Source: CAD feature listing. Evaluate the final solid. Frame: model axes, mm. A direction names the side the tool comes from. Coordinates: 2 decimals unless noted, no trailing zeros. Order: outer loops, then holes, each group sorted by start corner. A loop starts at its lowest first (then second) coordinate and runs counter-clockwise, first axis right, second up.
```python
from build123d import *
from build123d import SkipClean  # not in build123d's __all__

# Parameters (mm, degrees)
F0_R     = 2.5
F0_R_2   = 6.05
F1_DEPTH = 5
F2_W     = 7
F2_H     = 5


with BuildPart() as f1:
    # F0 (on Right) → F1 (new body)
    with BuildSketch(Plane.YZ):
        with BuildLine():
            ThreePointArc((6.7973084028, 29.3303630369), (0, 25), (-6.7973084028, 29.3303630369))
            Line((-6.7973084028, 29.3303630369), (-7.8035829138, 31.4883256898))
            ThreePointArc((-7.8035829138, 31.4883256898), (-9.3550783484, 32.9840034331), (-11.5089912382, 33.0536400519))
            ThreePointArc((-11.5089912382, 33.0536400519), (-13.3939201328, 32.3357836379), (-15.2343672744, 31.5105387727))
            ThreePointArc((-15.2343672744, 31.5105387727), (-16.7081731596, 29.9382518369), (-16.7476422276, 27.7835750194))
            Line((-16.7476422276, 27.7835750194), (-15.9332757327, 25.5461214635))
            ThreePointArc((-15.9332757327, 25.5461214635), (-17.6776695297, 17.6776695297), (-25.5461214635, 15.9332757327))
            Line((-25.5461214635, 15.9332757327), (-27.7835750194, 16.7476422276))
            ThreePointArc((-27.7835750194, 16.7476422276), (-29.9382518369, 16.7081731596), (-31.5105387727, 15.2343672744))
            ThreePointArc((-31.5105387727, 15.2343672744), (-32.3357836379, 13.3939201328), (-33.0536400519, 11.5089912382))
            ThreePointArc((-33.0536400519, 11.5089912382), (-32.9840034331, 9.3550783484), (-31.4883256898, 7.8035829138))
            Line((-31.4883256898, 7.8035829138), (-29.3303630369, 6.7973084028))
            ThreePointArc((-29.3303630369, 6.7973084028), (-25, 0), (-29.3303630369, -6.7973084028))
            Line((-29.3303630369, -6.7973084028), (-31.4883256898, -7.8035829138))
            ThreePointArc((-31.4883256898, -7.8035829138), (-32.9840034331, -9.3550783484), (-33.0536400519, -11.5089912382))
            ThreePointArc((-33.0536400519, -11.5089912382), (-32.3357836379, -13.3939201328), (-31.5105387727, -15.2343672744))
            ThreePointArc((-31.5105387727, -15.2343672744), (-29.9382518369, -16.7081731596), (-27.7835750194, -16.7476422276))
            Line((-27.7835750194, -16.7476422276), (-25.5461214635, -15.9332757327))
            ThreePointArc((-25.5461214635, -15.9332757327), (-17.6776695297, -17.6776695297), (-15.9332757327, -25.5461214635))
            Line((-15.9332757327, -25.5461214635), (-16.7476422276, -27.7835750194))
            ThreePointArc((-16.7476422276, -27.7835750194), (-16.7081731596, -29.9382518369), (-15.2343672744, -31.5105387727))
            ThreePointArc((-15.2343672744, -31.5105387727), (-13.3939201328, -32.3357836379), (-11.5089912382, -33.0536400519))
            ThreePointArc((-11.5089912382, -33.0536400519), (-9.3550783484, -32.9840034331), (-7.8035829138, -31.4883256898))
            Line((-7.8035829138, -31.4883256898), (-6.7973084028, -29.3303630369))
            ThreePointArc((-6.7973084028, -29.3303630369), (0, -25), (6.7973084028, -29.3303630369))
            Line((6.7973084028, -29.3303630369), (7.8035829138, -31.4883256898))
            ThreePointArc((7.8035829138, -31.4883256898), (9.3550783484, -32.9840034331), (11.5089912382, -33.0536400519))
            ThreePointArc((11.5089912382, -33.0536400519), (13.3939201328, -32.3357836379), (15.2343672744, -31.5105387727))
            ThreePointArc((15.2343672744, -31.5105387727), (16.7081731596, -29.9382518369), (16.7476422276, -27.7835750194))
            Line((16.7476422276, -27.7835750194), (15.9332757327, -25.5461214635))
            ThreePointArc((15.9332757327, -25.5461214635), (17.6776695297, -17.6776695297), (25.5461214635, -15.9332757327))
            Line((25.5461214635, -15.9332757327), (27.7835750194, -16.7476422276))
            ThreePointArc((27.7835750194, -16.7476422276), (29.9382518369, -16.7081731596), (31.5105387727, -15.2343672744))
            ThreePointArc((31.5105387727, -15.2343672744), (32.3357836379, -13.3939201328), (33.0536400519, -11.5089912382))
            ThreePointArc((33.0536400519, -11.5089912382), (32.9840034331, -9.3550783484), (31.4883256898, -7.8035829138))
            Line((31.4883256898, -7.8035829138), (29.3303630369, -6.7973084028))
            ThreePointArc((29.3303630369, -6.7973084028), (25, 0), (29.3303630369, 6.7973084028))
            Line((29.3303630369, 6.7973084028), (31.4883256898, 7.8035829138))
            ThreePointArc((31.4883256898, 7.8035829138), (32.9840034331, 9.3550783484), (33.0536400519, 11.5089912382))
            ThreePointArc((33.0536400519, 11.5089912382), (32.3357836379, 13.3939201328), (31.5105387727, 15.2343672744))
            ThreePointArc((31.5105387727, 15.2343672744), (29.9382518369, 16.7081731596), (27.7835750194, 16.7476422276))
            Line((27.7835750194, 16.7476422276), (25.5461214635, 15.9332757327))
            ThreePointArc((25.5461214635, 15.9332757327), (17.6776695297, 17.6776695297), (15.9332757327, 25.5461214635))
            Line((15.9332757327, 25.5461214635), (16.7476422276, 27.7835750194))
            ThreePointArc((16.7476422276, 27.7835750194), (16.7081731596, 29.9382518369), (15.2343672744, 31.5105387727))
            ThreePointArc((15.2343672744, 31.5105387727), (13.3939201328, 32.3357836379), (11.5089912382, 33.0536400519))
            ThreePointArc((11.5089912382, 33.0536400519), (9.3550783484, 32.9840034331), (7.8035829138, 31.4883256898))
            Line((7.8035829138, 31.4883256898), (6.7973084028, 29.3303630369))
        make_face()
        with Locations((-15.1554445662, -8.75)):
            Circle(F0_R, mode=Mode.SUBTRACT)
        with Locations((0, -17.5)):
            Circle(F0_R, mode=Mode.SUBTRACT)
        with Locations((15.1554445662, -8.75)):
            Circle(F0_R, mode=Mode.SUBTRACT)
        with Locations((-15.1554445662, 8.75)):
            Circle(F0_R, mode=Mode.SUBTRACT)
        Circle(F0_R_2, mode=Mode.SUBTRACT)
        with Locations((15.1554445662, 8.75)):
            Circle(F0_R, mode=Mode.SUBTRACT)
        with Locations((0, 17.5)):
            Circle(F0_R, mode=Mode.SUBTRACT)
    extrude(amount=F1_DEPTH)

    # F2 (on Front) → F3 (revolve)
    with BuildSketch(Plane.XZ):
        with Locations((-3.5, 8.55)):
            Rectangle(F2_W, F2_H)
    with SkipClean():  # cleaning this boolean's faces spoils the solid; the shape is the same uncleaned
        revolve(axis=Axis((9.7608398646, 0, 0), (1, 0, 0)))


solid = f1.part
```
1. Section query A-A, the plane y = -5. Output: boundary loops of the cut face in (x, z).
2. Section query D-D, the plane z = 23.5. Output: boundary loops of the cut face in (x, y), plus the area to 3 significant figures.
3. Draft query along Z for faces 1 (the cylindrical face through (2.46, -17.14, 7.23)), 2 (the cylindrical face through (2, 0, -25)), 3 (the flat face through (2.465, -26.649, 16.335)). Return one class per face: +Z half, -Z half, draft (parallel to the pull), parting line (faces both ways), or undercut.
4. Material intervals for line 1 along X through (y, z) = (-9.5, 8.5); line 2 along Z through (x, y) = (-5, 0); line 3 along Y through (x, z) = (1.75, 23), sorted ascending.
5. Section query B-B, the plane x = -1. Output: boundary loops of the cut face in (y, z), plus the area to 3 significant figures.
6. Contact query for flat-ended pins moving along their axis: P1, Ø6, axis at y = -15.16, z = 8.75, coming from the -X side; P2, Ø9.5, axis at y = 0, z = 0, coming from the -X side; P3, Ø3, axis at x = -5, y = -9.5, coming from the +Z side; P4, Ø2, axis at x = 2, y = 5, coming from the +Z side. Output: stop coordinate, or through.
7. Access query for faces 4 (the cylindrical face through (2.465, -13.368, 32.347)), 5 (the flat face through (2.465, 7.307, 30.424)), 6 (the cylindrical face through (2.46, 13.17, -10.27)), 7 (the flat face through (2.465, -7.307, -30.424)), 8 (the flat face through (2.465, 16.335, 26.649)). Directions: +Z, -Z, +X, -X, +Y, -Y. A direction counts if a zero-diameter tool reaches every point of the face in a straight line with its end or side. Return the directions, or none.
8. Section query C-C, the plane z = 8.75. Output: boundary loops of the cut face in (x, y).
Answer key:
1. outline: (-7, -9.85) - (0, -9.85) - (0, -26.91) - (5, -26.91) - (5, -3.41) - (-7, -3.41) - close; (-7, 3.41) - (5, 3.41) - (5, 26.91) - (0, 26.91) - (0, 9.85) - (-7, 9.85) - close
2. outline: (0, -15.5) - (5, -15.5) - (5, 15.5) - (0, 15.5) - close
2. area: 155 mm2
3. face 1: undercut
3. face 2: -Z half
3. face 3: +Z half
4. line 1: x = 0 to 5
4. line 2: z = -11.05 to -6.05, 6.05 to 11.05
4. line 3: y = -15.48 to 15.48
5. outline: circle Ø22.1 at (0, 0); hole circle Ø12.1 at (0, 0)
5. area: 269 mm2
6. P1: stops at x = 0
6. P2: passes through
6. P3: stops at z = 7.62
6. P4: stops at z = 28
7. face 4: +Z, +X, -X, -Y
7. face 5: +Z, +X, -X
7. face 6: +X, -X
7. face 7: -Z, +X, -X
7. face 8: +X, -X, +Y
8. outline: (-7, -6.75) - (0, -6.75) - (0, -12.66) - (5, -12.66) - (5, 12.66) - (0, 12.66) - (0, 6.75) - (-7, 6.75) - close; (0, -32.64) - (5, -32.64) - (5, -17.66) - (0, -17.66) - close; (0, 17.66) - (5, 17.66) - (5, 32.64) - (0, 32.64) - close
